Source: CAD feature listing. Evaluate the final solid. Frame: model axes, mm. A direction names the side the tool comes from. Round coordinates to 2 decimals unless told otherwise and drop trailing zeros. Write each loop counter-clockwise with the first axis right and the second up, starting at its lowest first coordinate (ties: lowest second). Pieces come first, ordered by that corner, then holes. Notation, with made-up numbers: (52.5, 52.5) -> (70.5, 52.5) arc R22 cw to (70.5, 64.5) -> close; hole circle Ø5 at (60, 66). An arc over 180 degrees is marked (long way). Put each result on its own line as item: value.
```python
from build123d import *

# Parameters (mm, degrees)
EXTRUDE_1_DEPTH            = 6
EXTRUDE_1_DEPTH_BACK       = 0.0001
SKETCH_1_W                 = 384.2
SKETCH_1_H                 = 517.4
SKETCH_2562_W              = 18
SKETCH_2562_H              = 6.2
EXTRUDE_2573_DEPTH         = 6
CUT_EXTRUDE_4_DEPTH        = 716.027083403
CUT_EXTRUDE_4_DEPTH_BACK   = 716.027083403
SKETCH_2698_W              = 17
SKETCH_2698_H              = 505.4
EXTRUDE_2764_DEPTH         = 6
SKETCH_2820_W              = 6.2
SKETCH_2820_H              = 18
EXTRUDE_2968_DEPTH         = 6
CUT_EXTRUDE_4_2_DEPTH      = 736.415052878
CUT_EXTRUDE_4_2_DEPTH_BACK = 736.415052878


with BuildPart() as part:
    # Эскиз1 → Бобышка-Вытянуть1 (new, two sides: drawn at the far end of the back side and taken through both)
    with BuildSketch(Plane.XY.offset(-EXTRUDE_1_DEPTH_BACK)):
        with Locations((472.1, -0.1)):
            Rectangle(SKETCH_1_W, SKETCH_1_H)
        Polygon((624.2, 179.571602285), (490.783243916, -0.1), (624.2, -179.771602285), align=None, mode=Mode.SUBTRACT)
        Polygon((615.81439814, 218.6), (472.1, 25.060620516), (328.38560186, 218.6), align=None, mode=Mode.SUBTRACT)
        Polygon((615.81439814, -218.8), (328.38560186, -218.8), (472.1, -25.260620516), align=None, mode=Mode.SUBTRACT)
        Polygon((320, 179.571602285), (320, -179.771602285), (453.416756084, -0.1), align=None, mode=Mode.SUBTRACT)
    extrude(amount=EXTRUDE_1_DEPTH + EXTRUDE_1_DEPTH_BACK)

    # Sketch 2562 → Extrude 2573 (add)
    with BuildSketch(Plane.XY):
        with Locations((335, -261.6)):
            Rectangle(SKETCH_2562_W, SKETCH_2562_H)
        with Locations((472.1, -261.6)):
            Rectangle(SKETCH_2562_W, SKETCH_2562_H)
        with Locations((609.2, -261.6)):
            Rectangle(SKETCH_2562_W, SKETCH_2562_H)
        with Locations((335, 261.4)):
            Rectangle(SKETCH_2562_W, SKETCH_2562_H)
        with Locations((472.1, 261.4)):
            Rectangle(SKETCH_2562_W, SKETCH_2562_H)
        with Locations((609.2, 261.4)):
            Rectangle(SKETCH_2562_W, SKETCH_2562_H)
    extrude(amount=EXTRUDE_2573_DEPTH)

    # Sketch 4 → Cut-Extrude 4 (cut, two sides: drawn at the far end of the back side and taken through both)
    with BuildSketch(Plane.XY.offset(-CUT_EXTRUDE_4_DEPTH_BACK)):
        Polygon((401.3, -259.8), (405.8, -259.8), (405.8, -250.3), (407.2, -250.3), (407.2, -246.9), (405.8, -246.9), (405.8, -243.8), (401.3, -243.8), (401.3, -246.9), (399.9, -246.9), (399.9, -250.3), (401.3, -250.3), align=None)
        Polygon((538.4, -259.8), (542.9, -259.8), (542.9, -250.3), (544.3, -250.3), (544.3, -246.9), (542.9, -246.9), (542.9, -243.8), (538.4, -243.8), (538.4, -246.9), (537, -246.9), (537, -250.3), (538.4, -250.3), align=None)
        Polygon((401.3, 259.6), (405.8, 259.6), (405.8, 250.1), (407.2, 250.1), (407.2, 246.7), (405.8, 246.7), (405.8, 243.6), (401.3, 243.6), (401.3, 246.7), (399.9, 246.7), (399.9, 250.1), (401.3, 250.1), align=None)
        Polygon((538.4, 259.6), (542.9, 259.6), (542.9, 250.1), (544.3, 250.1), (544.3, 246.7), (542.9, 246.7), (542.9, 243.6), (538.4, 243.6), (538.4, 246.7), (537, 246.7), (537, 250.1), (538.4, 250.1), align=None)
    extrude(amount=CUT_EXTRUDE_4_DEPTH + CUT_EXTRUDE_4_DEPTH_BACK, mode=Mode.SUBTRACT)

    # Sketch 2698 → Extrude 2764 (add)
    with BuildSketch(Plane.XY):
        with Locations((671.7, 5.9)):
            Rectangle(SKETCH_2698_W, SKETCH_2698_H)
    extrude(amount=EXTRUDE_2764_DEPTH)

    # Sketch 2820 → Extrude 2968 (add)
    with BuildSketch(Plane.XY):
        with Locations((683, -198.8)):
            Rectangle(SKETCH_2820_W, SKETCH_2820_H)
        with Locations((683, -0.1)):
            Rectangle(SKETCH_2820_W, SKETCH_2820_H)
        with Locations((683, 198.6)):
            Rectangle(SKETCH_2820_W, SKETCH_2820_H)
    extrude(amount=EXTRUDE_2968_DEPTH)

    # Sketch 4 2 → Cut-Extrude 4 2 (cut, two sides: drawn at the far end of the back side and taken through both)
    with BuildSketch(Plane.XY.offset(-CUT_EXTRUDE_4_2_DEPTH_BACK)):
        Polygon((681.2, -116.05), (681.2, -111.55), (671.7, -111.55), (671.7, -110.15), (668.3, -110.15), (668.3, -111.55), (665.2, -111.55), (665.2, -116.05), (668.3, -116.05), (668.3, -117.45), (671.7, -117.45), (671.7, -116.05), align=None)
        Polygon((681.2, 111.35), (681.2, 115.85), (671.7, 115.85), (671.7, 117.25), (668.3, 117.25), (668.3, 115.85), (665.2, 115.85), (665.2, 111.35), (668.3, 111.35), (668.3, 109.95), (671.7, 109.95), (671.7, 111.35), align=None)
    extrude(amount=CUT_EXTRUDE_4_2_DEPTH + CUT_EXTRUDE_4_2_DEPTH_BACK, mode=Mode.SUBTRACT)


solid = part.part
```
Q1. Pin query (flat end, axial travel): pin 1 (1.5 mm diameter, centred on y = -245, z = 4, fed in from +X); pin 2 (1.1 mm diameter, centred on x = 537.5, z = 2.5, fed in from -Y); pin 3 (1 mm diameter, centred on x = 352, z = 2, fed in from +Y). Return the tip coordinate at first contact, or that it passes through.
Ans:
pin 1: stops at x = 680.2
pin 2: stops at y = -258.8
pin 3: stops at y = 258.6
Q2. Reachability of faces 3 (the flat face through (480, 4, 6)), 4 (the flat face through (542.951, -120.676, 2.958)) from +Z, -Z, +X, -X, +Y, -Y: full face, straight path, thin tool, end or side. Return the list, or none.
Ans:
face 3: +Z, +X, -X, +Y, -Y
face 4: +Z, -Z
Q3. Draft query along Y for faces 1 (the flat face through (673, 9, 0)), 2 (the flat face through (399.237, -123.385, 2.958)). Return one class per face: +Y half, -Y half, draft (parallel to the pull), parting line (faces both ways), or undercut.
Ans:
face 1: draft
face 2: undercut
Q4. Material intervals for line 1 (X direction, y = -146.5, z = 1.5); line 2 (Y direction, x = 500, z = 3); line 3 (X direction, y = 139.5, z = 3), sorted ascending. Write a range as [from, to].
Ans:
line 1: x = [280, 320], [344.71, 382.07], [562.13, 599.49], [624.2, 680.2]
line 2: y = [-258.8, -218.8], [-62.83, -12.51], [12.31, 62.63], [218.6, 258.6]
line 3: x = [280, 320], [349.76, 387.12], [557.08, 594.44], [624.2, 680.2]
Q5. Cut plane A-A on x = 514. Output: boundary loops of the cut face in (y, z).
Ans:
outline: (-258.8, 0) -> (-218.8, 0) -> (-218.8, 6) -> (-258.8, 6) -> close; (-81.69, 0) -> (-31.37, 0) -> (-31.37, 6) -> (-81.69, 6) -> close; (31.17, 0) -> (81.49, 0) -> (81.49, 6) -> (31.17, 6) -> close; (218.6, 0) -> (258.6, 0) -> (258.6, 6) -> (218.6, 6) -> close
Q6. Cut plane D-D on x = 638. Output: boundary loops of the cut face in (y, z).
Ans:
outline: (-258.8, 0) -> (258.6, 0) -> (258.6, 6) -> (-258.8, 6) -> close
Q7. Cut plane B-B on y = -31.5. Give the number of separate pieces and of enclosed holes in the cut face, and give its area (3 significant figures).
Ans:
separate pieces: 4
enclosed holes: 0
area: 1,020 mm^2
